Part model, mm, in its own coordinate system. Face numbers are marked on the shaded views. Coordinates: 2 decimals unless noted, no trailing zeros. Loops run counter-clockwise (first coordinate to the right, second up) from the corner with the lowest first, then second, coordinate; pieces in that order, holes last.
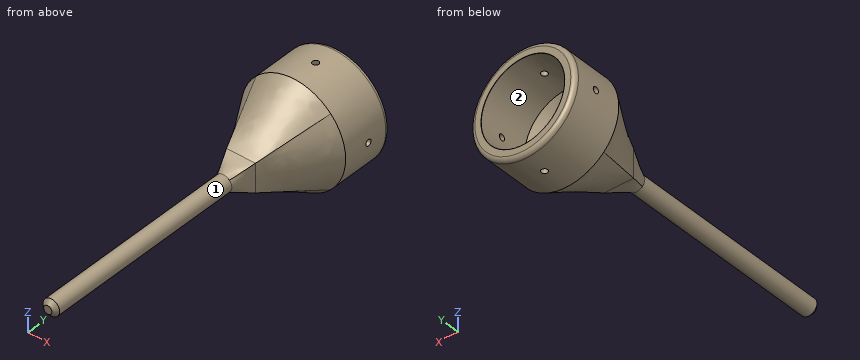
```python
from build123d import *

# Parameters (mm, degrees)
SKETCH1_R               = 3.98
BOSS_EXTRUDE1_DEPTH     = 85
SKETCH2_R               = 3.98
BOSS_EXTRUDE2_DEPTH     = 15.5
SKETCH5_W               = 13.94395882
SKETCH5_H               = 13.682539698
SKETCH7_W               = 13.94395882
SKETCH7_H               = 13.682539698
SKETCH8_R               = 20
CUT_EXTRUDE2_DEPTH      = 15.5
CUT_EXTRUDE2_DRAFT      = -36
SKETCH9_R               = 25
SKETCH9_R_2             = 20
BOSS_EXTRUDE3_DEPTH     = 25
SKETCH11_R              = 1.5
CUT_EXTRUDE3_DEPTH      = 30
CUT_EXTRUDE3_DEPTH_BACK = 30
SKETCH12_R              = 1.5
CUT_EXTRUDE4_DEPTH      = 30
CUT_EXTRUDE4_DEPTH_BACK = 30
FILLET2_R               = 2
FILLET3_R               = 0.1
CHAMFER1_SIZE           = 2


with BuildPart() as part:
    # Sketch1 → Boss-Extrude1 (new body)
    with BuildSketch(Plane(origin=(0, 0, 0), x_dir=(1, 0, 0), z_dir=(0, 1, 0))):
        with Locations(Location((0, 0, 0), (0, 0, 270))):
            Circle(SKETCH1_R)
    extrude(amount=BOSS_EXTRUDE1_DEPTH)

    # Sketch2 → Boss-Extrude2 (add)
    with BuildSketch(Plane(origin=(0, 85, 0), x_dir=(1, 0, 0), z_dir=(0, 1, 0))):
        with Locations(Location((0, 0, 0), (0, 0, 270))):
            Circle(SKETCH2_R)
    extrude(amount=BOSS_EXTRUDE2_DEPTH)

    # Sketch5 → Loft1 section 0
    with BuildSketch(Plane(origin=(0, 110.5, 0), x_dir=(1, 0, 0), z_dir=(0, 1, 0))):
        Rectangle(SKETCH5_W, SKETCH5_H)
    # Sketch4 for Loft1 → Loft1 section 1
    with BuildSketch(Plane(origin=(0, 100.5, 0), x_dir=(1, 0, 0), z_dir=(0, 1, 0))):
        with BuildLine():
            # circular arc as an exact rational Bezier (weights 1, cos(half-angle), 1)
            Bezier((-2.840788324, 2.787529677), (0, 5.682594209), (2.840788324, 2.787529677), weights=[1, 0.700384341, 1])
            Bezier((2.840788324, 2.787529677), (5.576057838, 0), (2.840788324, -2.787529677), weights=[1, 0.713765911, 1])
            Bezier((2.840788324, -2.787529677), (0, -5.682594209), (-2.840788324, -2.787529677), weights=[1, 0.700384341, 1])
            Bezier((-2.840788324, -2.787529677), (-5.576057838, 0), (-2.840788324, 2.787529677), weights=[1, 0.713765911, 1])
        make_face()
    loft()

    # Sketch6 for Loft2 → Loft2 section 0
    with BuildSketch(Plane(origin=(0, 140.5, 0), x_dir=(1, 0, 0), z_dir=(0, 1, 0))):
        with BuildLine():
            Bezier((-17.844147765, 17.509608521), (0, 35.694687248), (17.844147765, 17.509608521), weights=[1, 0.700384341, 1])
            Bezier((17.844147765, 17.509608521), (35.025488929, 0), (17.844147765, -17.509608521), weights=[1, 0.713765911, 1])
            Bezier((17.844147765, -17.509608521), (0, -35.694687248), (-17.844147765, -17.509608521), weights=[1, 0.700384341, 1])
            Bezier((-17.844147765, -17.509608521), (-35.025488929, 0), (-17.844147765, 17.509608521), weights=[1, 0.713765911, 1])
        make_face()
    # Sketch7 → Loft2 section 1
    with BuildSketch(Plane(origin=(0, 110.5, 0), x_dir=(1, 0, 0), z_dir=(0, 1, 0))):
        Rectangle(SKETCH7_W, SKETCH7_H)
    loft()


with BuildPart() as cut_extrude2_tool:
    # Sketch8 → Cut-Extrude2 (with draft: the straight prism first)
    with BuildSketch(Plane(origin=(0, 140.5, 0), x_dir=(1, 0, 0), z_dir=(0, 1, 0))):
        Circle(SKETCH8_R)
    extrude(amount=-CUT_EXTRUDE2_DEPTH)
    # Cut-Extrude2: the draft: its side faces are tilted about the plane it starts from
    cut_extrude2_sides = [cut_extrude2_tool.faces().sort_by_distance(p)[0] for p in [
        (-20, 132.75, 0),
    ]]
    draft(cut_extrude2_sides, Plane(origin=(0, 140.5, 0), x_dir=(1, 0, 0), z_dir=(0, 1, 0)), CUT_EXTRUDE2_DRAFT)


with BuildPart() as part_1:
    add(part.part)

    # Cut-Extrude2: cut by cut_extrude2_tool
    add(cut_extrude2_tool.part, mode=Mode.SUBTRACT)

    # Sketch9 → Boss-Extrude3 (add)
    with BuildSketch(Plane(origin=(0, 140.5, 0), x_dir=(1, 0, 0), z_dir=(0, 1, 0))):
        with Locations(Location((0, 0, 0), (0, 0, 44.457847859))):
            Circle(SKETCH9_R)
        with Locations(Location((0, 0, 0), (0, 0, 270))):
            Circle(SKETCH9_R_2, mode=Mode.SUBTRACT)
    extrude(amount=BOSS_EXTRUDE3_DEPTH)

    # Sketch11 → Cut-Extrude3 (cut, two sides)
    with BuildSketch(Plane(origin=(0, 0, 0), x_dir=(0, 0, -1), z_dir=(1, 0, 0))) as cut_extrude3_sk:
        with Locations(Location((0, 153.583337253, 0), (0, 0, 180))):
            Circle(SKETCH11_R)
    extrude(amount=CUT_EXTRUDE3_DEPTH, mode=Mode.SUBTRACT)
    extrude(cut_extrude3_sk.sketch, amount=-CUT_EXTRUDE3_DEPTH_BACK, mode=Mode.SUBTRACT)

    # Sketch12 → Cut-Extrude4 (cut, two sides)
    with BuildSketch(Plane.XY) as cut_extrude4_sk:
        with Locations(Location((0, 153.141524967, 0), (0, 0, 180))):
            Circle(SKETCH12_R)
    extrude(amount=CUT_EXTRUDE4_DEPTH, mode=Mode.SUBTRACT)
    extrude(cut_extrude4_sk.sketch, amount=-CUT_EXTRUDE4_DEPTH_BACK, mode=Mode.SUBTRACT)

    # Fillet2
    fillet2_edges = [part_1.edges().sort_by_distance(p)[0] for p in [
        (-17.844147764, 165.5, 17.509608521),
    ]]
    fillet(fillet2_edges, radius=FILLET2_R)

    # Fillet3
    fillet3_edges = [part_1.edges().sort_by_distance(p)[0] for p in [
        (0, 165.5, -20),
    ]]
    fillet(fillet3_edges, radius=FILLET3_R)

    # Chamfer1
    chamfer1_edges = [part_1.edges().sort_by_distance(p)[0] for p in [
        (0, 0, -3.98),
    ]]
    chamfer(chamfer1_edges, length=CHAMFER1_SIZE)


solid = part_1.part
```
Q1. Saw through at C-C (y = 64). List the corners of the cut face in (x, z), plus the area to 3 significant figures.
Q2. Probe line 1 (Z direction, x = 0, y = 149); line 2 (Y direction, x = 0, z = 21); line 3 (Z direction, x = -18, y = 141.5). List the from-to ranges inside material, lowest first.
Q3. Mould opens along X. For the marked faces 1 and 2 say: released by +X, released by -X, zero draft, split by the parting line, or undercut.
Q4. Saw through at A-A (x = 0). Count the separate pieces of the cut face and the enclosed holes in it, plus the area to 3 significant figures.
Q5. Drop flat-ended pins along their axis: P1, Ø6, axis at x = 7, z = -5, coming from the -Y side; P2, Ø5, axis at x = 14, z = 3, coming from the -Y side; P3, Ø5, axis at x = -7, y = 29.5, coming from the +Z side; P4, Ø14, axis at x = -1.5, z = -0.5, coming from the +Y side. Give the stop position or say it passes through.
Checked values:
1. outline: circle Ø7.96 at (0, 0)
1. area: 49.8 mm2
2. line 1: z = -25 to -20, 20 to 25
2. line 2: y = 133.89 to 151.64, 154.64 to 165.5
2. line 3: z = -17.35 to -8.72, 8.72 to 17.35
3. face 1: split by the parting line
3. face 2: undercut
4. separate pieces: 3
4. enclosed holes: 0
4. area: 1,630 mm2
5. P1: stops at y = 103.66
5. P2: stops at y = 118.31
5. P3: passes through
5. P4: stops at y = 125
